The listing builds one solid part. Answer for the finished solid, in the listing's coordinates (mm). Face numbers are marked on the shaded views. A direction names the side the tool comes from. Give positions to 0.01 mm unless a question says otherwise; leave off trailing zeros. Write each loop counter-clockwise with the first axis right and the second up, starting at its lowest first coordinate (ties: lowest second). Pieces come first, ordered by that corner, then holes.
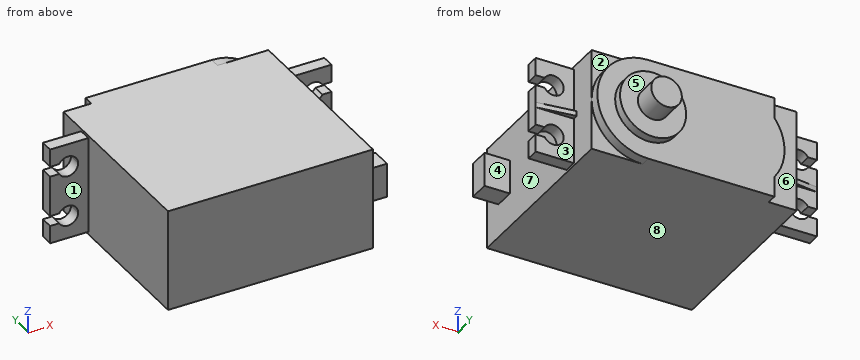
```python
from build123d import *

# Parameters (mm, degrees)
SKETCH1_W                = 40.3
SKETCH1_H                = 20
BOSS_EXTRUDE1_DEPTH      = 36.5
BOSS_EXTRUDE2_DEPTH      = 7.5
BOSS_EXTRUDE2_DEPTH_BACK = 47.8
SKETCH2_W                = 19
SKETCH2_H                = 2.5
CUT_EXTRUDE1_DEPTH       = 7.5
SKETCH5_W                = 7.5
SKETCH5_H                = 1
BOSS_EXTRUDE3_DEPTH      = 1
CUT_EXTRUDE2_DEPTH       = 1
BOSS_EXTRUDE4_DEPTH      = 2
SKETCH8_R                = 6.5
BOSS_EXTRUDE5_DEPTH      = 1.7
SKETCH9_R                = 3
BOSS_EXTRUDE6_DEPTH      = 4.7
SKETCH10_W               = 6.7
SKETCH10_H               = 4
BOSS_EXTRUDE7_DEPTH      = 5


with BuildPart() as part:
    # Sketch1 → Boss-Extrude1 (new body)
    with BuildSketch(Plane(origin=(0, 0, 0), x_dir=(1, 0, 0), z_dir=(0, 1, 0))):
        with Locations((20.15, 10)):
            Rectangle(SKETCH1_W, SKETCH1_H)
    extrude(amount=BOSS_EXTRUDE1_DEPTH)

    # Sketch2 → Boss-Extrude2 (add, two sides: drawn at the far end of the back side and taken through both)
    with BuildSketch(Plane.ZY.offset(-BOSS_EXTRUDE2_DEPTH_BACK)):
        with Locations((-10, 29.05)):
            Rectangle(SKETCH2_W, SKETCH2_H)
    extrude(amount=BOSS_EXTRUDE2_DEPTH + BOSS_EXTRUDE2_DEPTH_BACK)

    # Sketch3 → Cut-Extrude1 (cut)
    with BuildSketch(Plane(origin=(0, 30.3, 0), x_dir=(1, 0, 0), z_dir=(0, 1, 0))):
        with BuildLine():
            Line((-5.732050808, 14), (-5.5, 14))
            Line((-5.5, 14), (-5.5, 16))
            Line((-5.5, 16), (-5.732050808, 16))
            ThreePointArc((-5.732050808, 16), (-6, 15), (-5.732050808, 14))
        make_face()
        with BuildLine():
            Line((-5.5, 16), (-5.5, 14))
            Line((-5.5, 14), (-5.732050808, 14))
            ThreePointArc((-5.732050808, 14), (-3.48236191, 13.068148347), (-2, 15))
            ThreePointArc((-2, 15), (-3.48236191, 16.931851653), (-5.732050808, 16))
            Line((-5.732050808, 16), (-5.5, 16))
        make_face()
        with BuildLine():
            Line((-7.5, 14), (-5.732050808, 14))
            ThreePointArc((-5.732050808, 14), (-6, 15), (-5.732050808, 16))
            Line((-5.732050808, 16), (-7.5, 16))
            Line((-7.5, 16), (-7.5, 14))
        make_face()
        with BuildLine():
            Line((-7.5, 4), (-5.732050808, 4))
            ThreePointArc((-5.732050808, 4), (-6, 5), (-5.732050808, 6))
            Line((-5.732050808, 6), (-7.5, 6))
            Line((-7.5, 6), (-7.5, 4))
        make_face()
        with BuildLine():
            Line((-5.732050808, 4), (-5.5, 4))
            Line((-5.5, 4), (-5.5, 6))
            Line((-5.5, 6), (-5.732050808, 6))
            ThreePointArc((-5.732050808, 6), (-6, 5), (-5.732050808, 4))
        make_face()
        with BuildLine():
            Line((-5.5, 6), (-5.5, 4))
            Line((-5.5, 4), (-5.732050808, 4))
            ThreePointArc((-5.732050808, 4), (-3.48236191, 3.068148347), (-2, 5))
            ThreePointArc((-2, 5), (-3.48236191, 6.931851653), (-5.732050808, 6))
            Line((-5.732050808, 6), (-5.5, 6))
        make_face()
        with BuildLine():
            ThreePointArc((46.032050808, 16), (42.3, 15), (46.032050808, 14))
            Line((46.032050808, 14), (45.8, 14))
            Line((45.8, 14), (45.8, 16))
            Line((45.8, 16), (46.032050808, 16))
        make_face()
        with BuildLine():
            Line((45.8, 14), (46.032050808, 14))
            ThreePointArc((46.032050808, 14), (46.231851653, 14.48236191), (46.3, 15))
            ThreePointArc((46.3, 15), (46.231851653, 15.51763809), (46.032050808, 16))
            Line((46.032050808, 16), (45.8, 16))
            Line((45.8, 16), (45.8, 14))
        make_face()
        with BuildLine():
            Line((46.032050808, 14), (47.8, 14))
            Line((47.8, 14), (47.8, 16))
            Line((47.8, 16), (46.032050808, 16))
            ThreePointArc((46.032050808, 16), (46.231851653, 15.51763809), (46.3, 15))
            ThreePointArc((46.3, 15), (46.231851653, 14.48236191), (46.032050808, 14))
        make_face()
        with BuildLine():
            ThreePointArc((46.032050808, 6), (42.3, 5), (46.032050808, 4))
            Line((46.032050808, 4), (45.8, 4))
            Line((45.8, 4), (45.8, 6))
            Line((45.8, 6), (46.032050808, 6))
        make_face()
        with BuildLine():
            Line((45.8, 4), (46.032050808, 4))
            ThreePointArc((46.032050808, 4), (46.231851653, 4.48236191), (46.3, 5))
            ThreePointArc((46.3, 5), (46.231851653, 5.51763809), (46.032050808, 6))
            Line((46.032050808, 6), (45.8, 6))
            Line((45.8, 6), (45.8, 4))
        make_face()
        with BuildLine():
            Line((46.032050808, 4), (47.8, 4))
            Line((47.8, 4), (47.8, 6))
            Line((47.8, 6), (46.032050808, 6))
            ThreePointArc((46.032050808, 6), (46.231851653, 5.51763809), (46.3, 5))
            ThreePointArc((46.3, 5), (46.231851653, 4.48236191), (46.032050808, 4))
        make_face()
    extrude(amount=-CUT_EXTRUDE1_DEPTH, mode=Mode.SUBTRACT)

    # Sketch5 → Boss-Extrude3 (add)
    with BuildSketch(Plane(origin=(0, 30.3, 0), x_dir=(1, 0, 0), z_dir=(0, 1, 0))):
        with Locations((44.05, 10)):
            Rectangle(SKETCH5_W, SKETCH5_H)
        with Locations((-3.75, 10)):
            Rectangle(SKETCH5_W, SKETCH5_H)
    extrude(amount=BOSS_EXTRUDE3_DEPTH)

    # Sketch6 → Cut-Extrude2 (cut)
    with BuildSketch(Plane.XY.offset(-9.5)):
        Polygon((0, 31.3), (-7.5, 31.3), (-7.5, 30.3), align=None)
        Polygon((47.8, 30.3), (40.3, 31.3), (47.8, 31.3), align=None)
    extrude(amount=-CUT_EXTRUDE2_DEPTH, mode=Mode.SUBTRACT)

    # Sketch7 → Boss-Extrude4 (add)
    with BuildSketch(Plane(origin=(0, 36.5, 0), x_dir=(1, 0, 0), z_dir=(0, 1, 0))):
        with BuildLine():
            Line((30.3, 20), (13.5, 20))
            ThreePointArc((13.5, 20), (9.027864045, 18.94427191), (5.5, 16))
            Line((5.5, 16), (5.5, 4))
            ThreePointArc((5.5, 4), (9.027864045, 1.05572809), (13.5, 0))
            Line((13.5, 0), (30.3, 0))
            Line((30.3, 0), (30.3, 20))
        make_face()
        with BuildLine():
            Line((5.5, 4), (5.5, 16))
            ThreePointArc((5.5, 16), (3.5, 10), (5.5, 4))
        make_face()
        with BuildLine():
            Line((13.5, 20), (5.5, 20))
            Line((5.5, 20), (5.5, 16))
            ThreePointArc((5.5, 16), (9.027864045, 18.94427191), (13.5, 20))
        make_face()
        with BuildLine():
            ThreePointArc((13.5, 0), (9.027864045, 1.05572809), (5.5, 4))
            Line((5.5, 4), (5.5, 0))
            Line((5.5, 0), (13.5, 0))
        make_face()
        with BuildLine():
            ThreePointArc((30.3, 20), (40.3, 10), (30.3, 0))
            Line((30.3, 0), (30.3, 20))
        make_face()
    extrude(amount=BOSS_EXTRUDE4_DEPTH)

    # Sketch8 → Boss-Extrude5 (add)
    with BuildSketch(Plane(origin=(0, 38.5, 0), x_dir=(1, 0, 0), z_dir=(0, 1, 0))):
        with Locations(Location((30.3, 10, 0), (0, 0, 270))):
            Circle(SKETCH8_R)
    extrude(amount=BOSS_EXTRUDE5_DEPTH)

    # Sketch9 → Boss-Extrude6 (add)
    with BuildSketch(Plane(origin=(0, 40.2, 0), x_dir=(1, 0, 0), z_dir=(0, 1, 0))):
        with Locations(Location((30.3, 10, 0), (0, 0, 270))):
            Circle(SKETCH9_R)
    extrude(amount=BOSS_EXTRUDE6_DEPTH)

    # Sketch10 → Boss-Extrude7 (add)
    with BuildSketch(Plane(origin=(40.3, 0, 0), x_dir=(0, 0, -1), z_dir=(1, 0, 0))):
        with Locations((10, 6)):
            Rectangle(SKETCH10_W, SKETCH10_H)
    extrude(amount=BOSS_EXTRUDE7_DEPTH)


solid = part.part
```
Item 1: A cutting plane is placed at C-C, the plane y = 28.5. Give the vertices of the cut face in (x, z).
Conclusion:
outline: (-7.5, -19.5) - (0, -19.5) - (0, -20) - (40.3, -20) - (40.3, -19.5) - (47.8, -19.5) - (47.8, -16) - (46.03, -16) arc R2 cw (long way) to (46.03, -14) - (47.8, -14) - (47.8, -6) - (46.03, -6) arc R2 cw (long way) to (46.03, -4) - (47.8, -4) - (47.8, -0.5) - (40.3, -0.5) - (40.3, 0) - (0, 0) - (0, -0.5) - (-7.5, -0.5) - (-7.5, -4) - (-5.73, -4) arc R2 cw (long way) to (-5.73, -6) - (-7.5, -6) - (-7.5, -14) - (-5.73, -14) arc R2 cw (long way) to (-5.73, -16) - (-7.5, -16) - close
Item 2: Determine the mould class of the marked faces 6, 7 and 8 for opening direction Y: pulls with the +Y half, pulls with the -Y half, needs draft (parallel to the pull), parting line crosses it, or undercut.
Conclusion:
face 6: pulls with the +Y half
face 7: undercut
face 8: needs draft
Item 3: A cutting plane is placed at A-A, the plane y = 6.5. Give the vertices of the cut face in (x, z).
Conclusion:
outline: (0, -20) - (40.3, -20) - (40.3, -13.35) - (45.3, -13.35) - (45.3, -6.65) - (40.3, -6.65) - (40.3, 0) - (0, 0) - close
Item 4: Which of the six approach directions +Z, -Z, +X, -X, +Y, -Y give full straight-line access (tool end or side, diameter ignored) to the marked faces 1, 2, 3, 4 and 5?
Conclusion:
face 1: +Z, -Z, -X, -Y
face 2: +Z, +X, +Y
face 3: -Z, +X, +Y
face 4: +Z, -Z, +X
face 5: +Y
Item 5: A cutting plane is placed at B-B, the plane x = -3.5. Give the vertices of the cut face in (y, z), plus the area to 3 significant figures.
Conclusion:
outline: (27.8, -19.5) - (30.3, -19.5) - (30.3, -16.94) - (27.8, -16.94) - close; (27.8, -13.06) - (30.3, -13.06) - (30.3, -10.5) - (30.83, -10.5) - (30.83, -9.5) - (30.3, -9.5) - (30.3, -6.94) - (27.8, -6.94) - close; (27.8, -3.06) - (30.3, -3.06) - (30.3, -0.5) - (27.8, -0.5) - close
area: 28.7 mm2
Item 6: Each of these flat-tipped pins is pushed along its axis until it touches: P1, Ø8, axis at y = 13, z = -9.5, coming from the -X side; P2, Ø2, axis at x = -4.5, y = 29.5, coming from the -Z side; P3, Ø3.5, axis at x = 44.3, z = -5, coming from the +Y side. Where does it stop, or does it pass through?
Conclusion:
P1: stops at x = 0
P2: stops at z = -19.5
P3: stops at y = 8
Item 7: Consider probe 1 along Z at (x, y) = (44, 29); probe 2 along X at (y, z) = (27.5, -13.5); probe 3 along Y at (x, z) = (24, -13.5). Determine where each line is inside the solid, lowest interval first.
Conclusion:
probe 1: z = -19.5 to -16.98, -13.02 to -6.98, -3.02 to -0.5
probe 2: x = 0 to 40.3
probe 3: y = 0 to 38.5
Item 8: A cutting plane is placed at D-D, the plane y = 13.5. Give the vertices of the cut face in (x, z), plus the area to 3 significant figures.
Conclusion:
outline: (0, -20) - (40.3, -20) - (40.3, 0) - (0, 0) - close
area: 806 mm2
